Input: part model. Units: mm. Frame: model coordinates. A direction names the side the tool comes from. Coordinates: 2 decimals unless noted, no trailing zeros. Loops run counter-clockwise (first coordinate to the right, second up) from the corner with the lowest first, then second, coordinate; pieces in that order, holes last. Notation, with made-up numbers: (74.5, 27.25) -> (80.5, 27.25) arc R12 cw to (80.5, 34.25) -> close; hole circle Ø11 at (21.25, 2). An arc over 180 degrees is marked (long way). Answer as a JSON object with one key per item and string values.
from build123d import *

# Parameters (mm, degrees)
F1_DEPTH = 50
F2_R     = 24.99999
F3_R     = 9
F5_DEPTH = 60.001
F6_R     = 9
F7_DEPTH = 25.4


# Not quite as in the source:
# - a fillet or chamfer is up to 0.001 mm smaller than in the source, because OpenCascade refuses the exact size


with BuildPart() as f1:
    # F0 (on Front) → F1 (new body)
    with BuildSketch(Plane.XZ):
        Polygon((-110, 0), (-49, 0), (-49, 22), (0, 22), (0, 38), (-49, 38), (-49, 60), (-110, 60), (-110, 45), (-61, 45), (-61, 15), (-110, 15), align=None)
    extrude(amount=F1_DEPTH)

    # F2 (radius 25 in the source; OpenCascade refuses exactly that, so slightly less here)
    f2_edges = [f1.edges().sort_by_distance(p)[0] for p in [
        (-110, -50, 52.5),
        (-110, -50, 7.5),
        (-110, 0, 52.5),
        (-110, 0, 7.5),
        (0, -50, 30),
        (0, 0, 30),
    ]]
    fillet(f2_edges, radius=F2_R)

    # F3 (on face) → F5 (cut, through all)
    with BuildSketch(Plane(origin=(0, 0, 0), x_dir=(1, 0, 0), z_dir=(0, 0, -1))):
        with Locations((-85, 25)):
            Circle(F3_R)
    extrude(amount=-F5_DEPTH, mode=Mode.SUBTRACT)

    # F6 (on face) → F7 (cut)
    with BuildSketch(Plane(origin=(0, 0, 22), x_dir=(1, 0, 0), z_dir=(0, 0, -1))):
        with Locations((-25, 24.9226680556)):
            Circle(F6_R)
    extrude(amount=-F7_DEPTH, mode=Mode.SUBTRACT)


solid = f1.part
1. Access query for faces 4 (the face through (-49, -25, 49)), 5 (the face through (-75, -25, 45)), 6 (the face through (-49, -25, 11)), 7 (the face through (-73, -25, 0)). Directions: +Z, -Z, +X, -X, +Y, -Y. A direction counts if a zero-diameter tool reaches every point of the face in a straight line with its end or side. Return the directions, or none.
Reply:
{"face 4": "+Z, +X, +Y, -Y", "face 5": "-X, +Y, -Y", "face 6": "-Z, +X, +Y, -Y", "face 7": "-Z, +X, -X, +Y, -Y"}
2. Line query: line 1 along Y through (x, z) = (-25, 29); line 2 along Z through (x, y) = (-93, -11.5); line 3 along Y through (x, z) = (-85, 10). Output: solid intervals per line, ascending.
Reply:
{"line 1": "y = -50 to -33.92, -15.92 to 0", "line 2": "z = 0 to 15, 45 to 60", "line 3": "y = -50 to -34, -16 to 0"}
3. Mould query, pull axis X, two halves, no side actions, for faces 1 (the face through (-36, -25, 22)), 2 (the face through (-76.416, -27.703, 7.395)), 3 (the face through (-61, -25, 30)). Classes: pulls with the +X half, pulls with the -X half, needs draft (parallel to the pull), parting line crosses it, or undercut.
Reply:
{"face 1": "needs draft", "face 2": "undercut", "face 3": "pulls with the -X half"}
4. Pin query (flat end, axial travel): P1, Ø23.5, axis at x = -25, y = -24.92, coming from the +Z side; P2, Ø8, axis at y = -24.5, z = 8, coming from the -X side; P3, Ø11, axis at y = -26, z = 11, coming from the +X side; P4, Ø24.5, axis at x = -31, y = -22.5, coming from the -Z side. Return the tip coordinate at first contact, or that it passes through.
Reply:
{"P1": "stops at z = 38", "P2": "stops at x = -110", "P3": "stops at x = -49", "P4": "stops at z = 22"}
5. Section query B-B (x = -32.5). Return loops of the section in (y, z).
Reply:
{"outline": "(-50, 22) -> (-29.9, 22) -> (-29.9, 38) -> (-50, 38) -> close; (-19.95, 22) -> (0, 22) -> (0, 38) -> (-19.95, 38) -> close"}
6. Section query D-D (y = -46). Return loops of the section in (x, z).
Reply:
{"outline": "(-98.56, 0) -> (-49, 0) -> (-49, 22) -> (-11.44, 22) -> (-11.44, 38) -> (-49, 38) -> (-49, 60) -> (-98.56, 60) -> (-98.56, 45) -> (-61, 45) -> (-61, 15) -> (-98.56, 15) -> close"}
7. Section query C-C (y = -26.5). Return loops of the section in (x, z).
Reply:
{"outline": "(-109.95, 0) -> (-93.87, 0) -> (-93.87, 15) -> (-109.95, 15) -> close; (-109.95, 45) -> (-93.87, 45) -> (-93.87, 60) -> (-109.95, 60) -> close; (-76.13, 0) -> (-49, 0) -> (-49, 22) -> (-33.86, 22) -> (-33.86, 38) -> (-49, 38) -> (-49, 60) -> (-76.13, 60) -> (-76.13, 45) -> (-61, 45) -> (-61, 15) -> (-76.13, 15) -> close; (-16.14, 22) -> (-0.05, 22) -> (-0.05, 38) -> (-16.14, 38) -> close"}
